Source: CAD feature listing. Evaluate the final solid. Frame: model axes, mm. Face numbers are marked on the shaded views. A direction names the side the tool comes from. Round coordinates to 2 decimals unless told otherwise and drop trailing zeros. Loops run counter-clockwise (first coordinate to the right, second up) from the corner with the lowest first, then second, coordinate; pieces in that order, holes last. Notation, with made-up numbers: (54, -18) - (102, -18) arc R15 ccw to (102, 3) - close; hole circle Ø6 at (-10, 74). An arc over 180 degrees is marked (long way). Write item = value, one per line. Start each with the question number.
from build123d import *

# Parameters (mm, degrees)
BOSS_EXTRUDE1_DEPTH = 1.8


with BuildPart() as part:
    # Sketch1 → Boss-Extrude1 (new body)
    with BuildSketch(Plane(origin=(0, 0, 0), x_dir=(1, 0, 0), z_dir=(0, 1, 0))):
        with BuildLine():
            Line((-2.35, -2.85), (-2.55, -2.85))
            ThreePointArc((-2.55, -2.85), (-3.05, -3.35), (-2.55, -3.85))
            Line((-2.55, -3.85), (-1.35, -3.85))
            Line((-1.35, -3.85), (-1.35, -0.85))
            Line((-1.35, -0.85), (1.35, -0.85))
            Line((1.35, -0.85), (1.35, -3.85))
            Line((1.35, -3.85), (2.55, -3.85))
            ThreePointArc((2.55, -3.85), (3.05, -3.35), (2.55, -2.85))
            Line((2.55, -2.85), (2.35, -2.85))
            Line((2.35, -2.85), (2.35, 2.85))
            Line((2.35, 2.85), (2.55, 2.85))
            ThreePointArc((2.55, 2.85), (3.05, 3.35), (2.55, 3.85))
            Line((2.55, 3.85), (1.35, 3.85))
            Line((1.35, 3.85), (1.35, 0.85))
            Line((1.35, 0.85), (-1.35, 0.85))
            Line((-1.35, 0.85), (-1.35, 3.85))
            Line((-1.35, 3.85), (-2.55, 3.85))
            ThreePointArc((-2.55, 3.85), (-3.05, 3.35), (-2.55, 2.85))
            Line((-2.55, 2.85), (-2.35, 2.85))
            Line((-2.35, 2.85), (-2.35, -2.85))
        make_face()
    extrude(amount=BOSS_EXTRUDE1_DEPTH)


solid = part.part
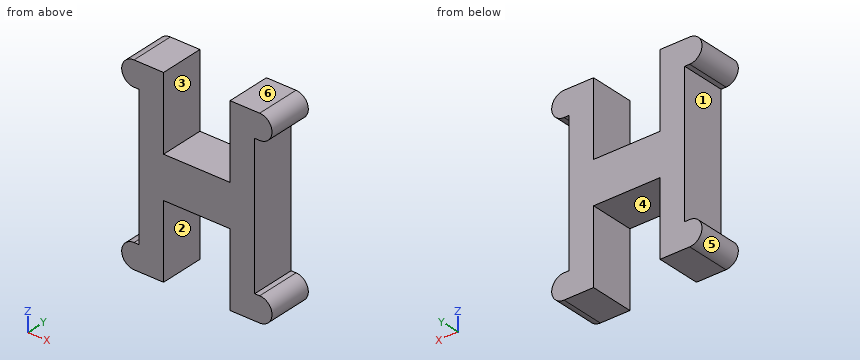
(1) Cut plane A-A (z = 2.25). Output: boundary loops of the cut face in (x, y).
(2) Cut plane D-D (x = -0.25). Output: boundary loops of the cut face in (y, z), and give its area (3 significant figures).
(3) Material intervals for line 1 along Z through (x, y) = (-2.5, 0.9); line 2 along X through (y, z) = (1.6, -2.75); line 3 along X through (y, z) = (0.4, 0.75), sorted ascending. Write a range as from..to.
(4) Access query for the marked faces 1, 2 and 3. Directions: +Z, -Z, +X, -X, +Y, -Y. A direction counts if a zero-diameter tool reaches every point of the face in a straight line with its end or side. Return the directions, or none.
(5) Pin query (flat end, axial travel): P1, Ø0.5, axis at y = 0.5, z = -3, coming from the -X side; P2, Ø1, axis at y = 0, z = 0, coming from the +X side; P3, Ø0.9, axis at x = 0, y = 0.5, coming from the +Z side; P4, Ø2, axis at x = 1, z = -3, coming from the +Y side. Return the tip coordinate at first contact, or that it passes through.
(6) Cut plane C-C (z = 3.35). Output: boundary loops of the cut face in (x, y).
(7) Mould query, pull axis X, two halves, no side actions, for the marked faces 4, 5 and 6. Classes: +X half, -X half, draft (parallel to the pull), parting line (faces both ways), or undercut.
(8) Cut plane B-B (y = 1.65). Output: boundary loops of the cut face in (x, z).
Solution:
q1.outline = (-2.35, 0) - (-1.35, 0) - (-1.35, 1.8) - (-2.35, 1.8) - close; (1.35, 0) - (2.35, 0) - (2.35, 1.8) - (1.35, 1.8) - close
q2.outline = (0, -0.85) - (1.8, -0.85) - (1.8, 0.85) - (0, 0.85) - close
q2.area = 3.06 mm^2
q3.line_1 = -3.85..-2.85, 2.85..3.85
q3.line_2 = -2.35..-1.35, 1.35..2.35
q3.line_3 = -2.35..2.35
q4.face_1 = -X, +Y, -Y
q4.face_2 = -Z, +Y, -Y
q4.face_3 = +Z, +Y, -Y
q5.P1 = -3.04
q5.P2 = 2.35
q5.P3 = 0.85
q5.P4 = 1.8
q6.outline = (-3.05, 0) - (-1.35, 0) - (-1.35, 1.8) - (-3.05, 1.8) - close; (1.35, 0) - (3.05, 0) - (3.05, 1.8) - (1.35, 1.8) - close
q7.face_4 = undercut
q7.face_5 = -X half
q7.face_6 = draft
q8.outline = (-2.55, -3.85) - (-1.35, -3.85) - (-1.35, -0.85) - (1.35, -0.85) - (1.35, -3.85) - (2.55, -3.85) arc R0.5 ccw to (2.55, -2.85) - (2.35, -2.85) - (2.35, 2.85) - (2.55, 2.85) arc R0.5 ccw to (2.55, 3.85) - (1.35, 3.85) - (1.35, 0.85) - (-1.35, 0.85) - (-1.35, 3.85) - (-2.55, 3.85) arc R0.5 ccw to (-2.55, 2.85) - (-2.35, 2.85) - (-2.35, -2.85) - (-2.55, -2.85) arc R0.5 ccw to start
